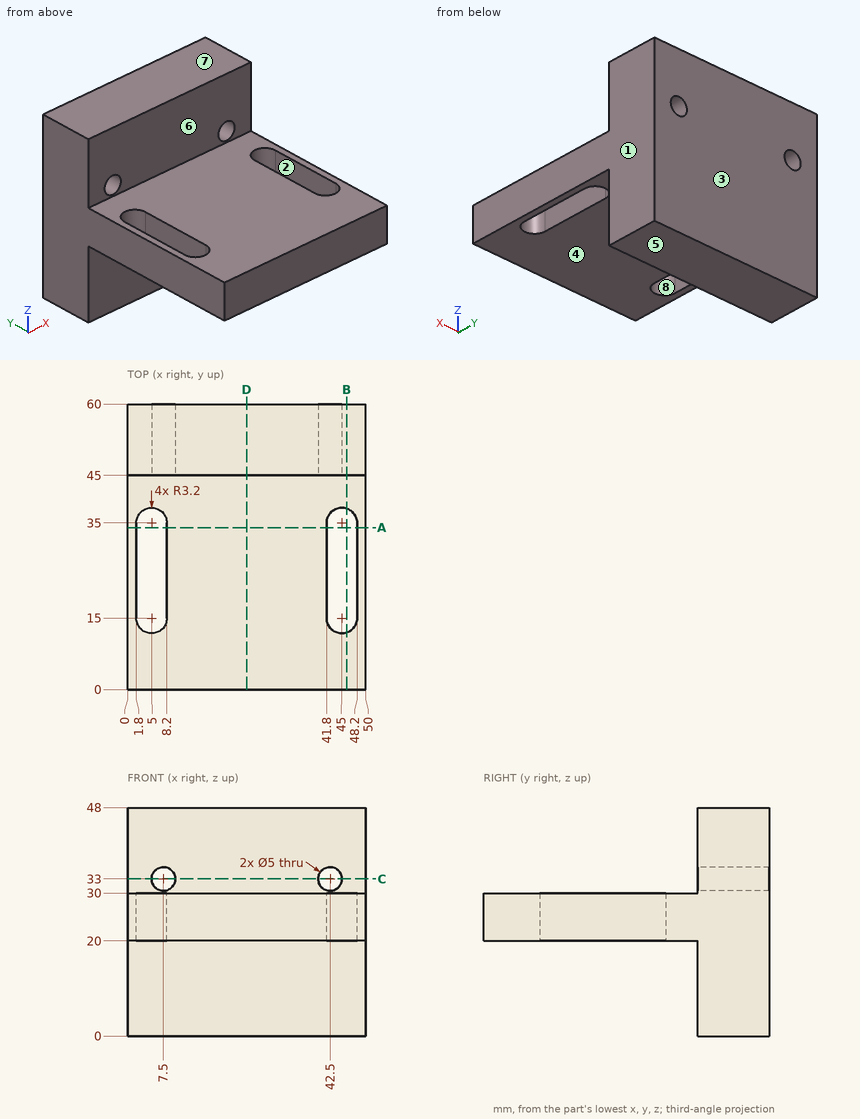
Part print with two shaded views. Sizes in mm from the minimum x, y, z corner. A direction names the side the tool comes from. Round coordinates to 2 decimals unless told otherwise and drop trailing zeros. Order: outer loops, then holes, each group sorted by start corner. A loop starts at its lowest first (then second) coordinate and runs counter-clockwise, first axis right, second up. Notation, with made-up numbers: (36.5, 20) - (52.5, 20) arc R26 cw to (52.5, 50) - close; hole circle Ø6 at (79.25, 53.25). An arc over 180 degrees is marked (long way). Return JSON: item names as keys, results as strings.
(1) Cut at A-A (y = 34). Give the cut face in (x, z), then the cut area to 3 significant figures.
Answer key:
{"outline": "(0, 20) - (1.8, 20) - (1.8, 30) - (0, 30) - close; (8.2, 20) - (41.8, 20) - (41.8, 30) - (8.2, 30) - close; (48.2, 20) - (50, 20) - (50, 30) - (48.2, 30) - close", "area": "372 mm^2"}
(2) Cut at B-B (x = 46). Give the cut face in (y, z), then the cut area to 3 significant figures.
Answer key:
{"outline": "(0, 20) - (11.96, 20) - (11.96, 30) - (0, 30) - close; (38.04, 20) - (45, 20) - (45, 0) - (60, 0) - (60, 48) - (45, 48) - (45, 30) - (38.04, 30) - close", "area": "909 mm^2"}
(3) Tool access for the marked faces 4, 5, 6, 7 and 8: list every direction of +Z, -Z, +X, -X, +Y, -Y with a clear straight run to the whole face (end or side of a thin tool).
Answer key:
{"face 4": "-Z, +X, -X, -Y", "face 5": "-Z, +X, -X, +Y, -Y", "face 6": "+Z, +X, -X, -Y", "face 7": "+Z, +X, -X, +Y, -Y", "face 8": "+Z, -Z"}
(4) Cut at C-C (z = 33). Give the cut face in (x, y), then the cut area to 3 significant figures.
Answer key:
{"outline": "(0, 45) - (5, 45) - (5, 60) - (0, 60) - close; (10, 45) - (40, 45) - (40, 60) - (10, 60) - close; (45, 45) - (50, 45) - (50, 60) - (45, 60) - close", "area": "600 mm^2"}
(5) Pull direction Y, two halves, no side cores. Call the marked faces 1, 2 and 3: +Y half, -Y half, draft (parallel to the pull), parting line (faces both ways), or undercut.
Answer key:
{"face 1": "draft", "face 2": "undercut", "face 3": "+Y half"}
(6) Pin check, flat tips, straight feed: pin 1 Ø6 at (x, z) = (21.5, 5.5) entering from -Y; pin 2 Ø12 at (x, y) = (24, 34.5) entering from +Z; pin 3 Ø12 at (x, y) = (34.5, 20.5) entering from -Z. Stop position of each tip, or through.
Answer key:
{"pin 1": "stops at y = 45", "pin 2": "stops at z = 30", "pin 3": "stops at z = 20"}
(7) Cut at D-D (x = 25). Give the cut face in (y, z).
Answer key:
{"outline": "(0, 20) - (45, 20) - (45, 0) - (60, 0) - (60, 48) - (45, 48) - (45, 30) - (0, 30) - close"}
(8) Wall check: probe 1 along X at (y, z) = (51.25, 33); probe 2 along Z at (x, y) = (42.5, 51); probe 3 along X at (y, z) = (46.5, 34.5). Give the ranges that are in metal, low to high. Write a range as from..to.
Answer key:
{"probe 1": "x = 0..5, 10..40, 45..50", "probe 2": "z = 0..30.5, 35.5..48", "probe 3": "x = 0..5.5, 9.5..40.5, 44.5..50"}
